For this review, take the finished solid that the model builds, in its own axes (mm). A direction names the side the tool comes from. Round coordinates to 2 decimals unless told otherwise and drop trailing zeros. Write each loop counter-clockwise with the first axis right and the second up, starting at its lowest first coordinate (ties: lowest second). Pieces come first, ordered by that corner, then holes. Notation, with made-up numbers: (20.5, 81.5) - (79.5, 81.5) arc R29 cw to (79.5, 116.5) - close; hole circle Ø7 at (81, 61). An arc over 180 degrees is marked (long way). Answer in a Markdown table with one row per item. Add a question column.
from build123d import *

# Parameters (mm, degrees)
SKETCH1_W                  = 120
SKETCH1_H                  = 80
BOSS_EXTRUDE1_DEPTH        = 15
SKETCH2_R                  = 33
BOSS_EXTRUDE2_DEPTH        = 48
BOSS_EXTRUDE3_DEPTH        = 15
SKETCH10_R                 = 21
CUT_EXTRUDE1_DEPTH         = 48
SKETCH11_R                 = 16.5
CUT_EXTRUDE2_DEPTH         = 15
M12X1_5_TAPPED_HOLE1_D     = 10.5
M12X1_5_TAPPED_HOLE1_DEPTH = 15
FILLET2_R                  = 2
FILLET3_R                  = 10


with BuildPart() as part:
    # Sketch1 → Boss-Extrude1 (new body)
    with BuildSketch(Plane(origin=(0, 0, 0), x_dir=(1, 0, 0), z_dir=(0, 1, 0))):
        Rectangle(SKETCH1_W, SKETCH1_H)
    extrude(amount=BOSS_EXTRUDE1_DEPTH)

    # Sketch2 → Boss-Extrude2 (add)
    with BuildSketch(Plane(origin=(0, 0, 0), x_dir=(1, 0, 0), z_dir=(0, 1, 0))):
        with Locations(Location((0, 0, 0), (0, 0, 270))):
            Circle(SKETCH2_R)
    extrude(amount=BOSS_EXTRUDE2_DEPTH)

    # Sketch3 → Boss-Extrude3 (add)
    with BuildSketch(Plane(origin=(0, 48, 0), x_dir=(1, 0, 0), z_dir=(0, 1, 0))):
        with BuildLine():
            ThreePointArc((-56.391046334, 10.447445772), (0, 36), (56.391046334, 10.447445772))
            ThreePointArc((56.391046334, 10.447445772), (59.733253975, 0), (56.391046334, -10.447445772))
            ThreePointArc((56.391046334, -10.447445772), (0, -36), (-56.391046334, -10.447445772))
            ThreePointArc((-56.391046334, -10.447445772), (-59.733253975, 0), (-56.391046334, 10.447445772))
        make_face()
    extrude(amount=BOSS_EXTRUDE3_DEPTH)

    # Sketch10 → Cut-Extrude1 (cut)
    with BuildSketch(Plane(origin=(0, 63, 0), x_dir=(1, 0, 0), z_dir=(0, 1, 0))):
        with Locations(Location((0, 0, 0), (0, 0, 270))):
            Circle(SKETCH10_R)
    extrude(amount=-CUT_EXTRUDE1_DEPTH, mode=Mode.SUBTRACT)

    # Sketch11 → Cut-Extrude2 (cut)
    with BuildSketch(Plane(origin=(0, 15, 0), x_dir=(1, 0, 0), z_dir=(0, 1, 0))):
        with Locations(Location((0, 0, 0), (0, 0, 270))):
            Circle(SKETCH11_R)
    extrude(amount=-CUT_EXTRUDE2_DEPTH, mode=Mode.SUBTRACT)

    # M12x1.5 Tapped Hole1
    with Locations(Plane(origin=(-42, 63, 0), x_dir=(0, 0, 1), z_dir=(0, 1, 0))):
        with Locations((0, 0), (0, 84)):
            Hole(M12X1_5_TAPPED_HOLE1_D / 2, depth=M12X1_5_TAPPED_HOLE1_DEPTH)

    # Fillet2
    fillet2_edges = [part.edges().sort_by_distance(p)[0] for p in [
        (0, 15, -33),
        (0, 48, -33),
    ]]
    fillet(fillet2_edges, radius=FILLET2_R)

    # Fillet3
    fillet3_edges = [part.edges().sort_by_distance(p)[0] for p in [
        (60, 7.5, 40),
        (-60, 7.5, 40),
        (-60, 7.5, -40),
        (60, 7.5, -40),
    ]]
    fillet(fillet3_edges, radius=FILLET3_R)


solid = part.part
Q1. To check wall thickness, follow probe 1 along X at (y, z) = (42.5, 0); probe 2 along Y at (x, z) = (48, 4); probe 3 along X at (y, z) = (9.25, 0). State the ranges of each line that lie inside material, in increasing order.
Q2. Tool access review of faces 5 (the face through (-11, 15, -13)), 6 (the face through (0.893, 55.395, 35.995)), 7 (the face through (59.733, 55.395, -0.156)): name each direction out of +Z, -Z, +X, -X, +Y, -Y from which nothing blocks a thin tool from reaching the whole face with its end or side.
Q3. Add section D-D on z = 0.5. Count the separate pieces of the cut face and the enclosed holes in it, then the cut area to 3 significant figures.
Q4. Insertion check: pin 1 Ø6 at (x, y) = (45.5, 52.5) entering from -Z; pin 2 Ø5 at (y, z) = (52.5, 16) entering from +X; pin 3 Ø6.5 at (x, z) = (-42, 0) entering from +Y. Each pin has a flat end and moves straight along its axis. Give the tip position at first contact, or say it passes through.
Q5. Add section B-B on x = -42. State the section outline as (y, z) points, then the cut area to 3 significant figures.
Q6. Add section A-A on x = 0. State the section outline as (y, z) points, then the cut area to 3 significant figures.
Q7. Draft analysis for pull direction Z (two halves, no side actions). For faces 1 (the face through (-36.795, 55.395, 0.683)), 2 (the face through (-1, 7, 40)), 3 (the face through (6.31, 39.34, 20.03)), 4 (the face through (-57.15, 7.6, -36.99)), state which applies: released by +Z, released by -Z, zero draft, split by the parting line, or undercut.
Q8. Add section C-C on y = 20. State the section outline as (x, z) points, then the cut area to 3 significant figures.
Answer sheet:
| question | item | result |
|---|---|---|
| 1 | probe 1 | x = -33 to -21, 21 to 33 |
| 1 | probe 2 | y = 0 to 15, 48 to 63 |
| 1 | probe 3 | x = -60 to -16.5, 16.5 to 60 |
| 2 | face 5 | +Y |
| 2 | face 6 | +Z, +Y |
| 2 | face 7 | +X, +Y |
| 3 | separate pieces | 4 |
| 3 | enclosed holes | 0 |
| 3 | area | 2,950 mm² |
| 4 | pin 1 | stops at z = -22.8 |
| 4 | pin 2 | stops at x = 53.56 |
| 4 | pin 3 | stops at y = 15 |
| 5 | outline | (0, -40) - (15, -40) - (15, 40) - (0, 40) - close; (48, -23.14) - (63, -23.14) - (63, -5.25) - (48, -5.25) - close; (48, 5.25) - (63, 5.25) - (63, 23.14) - (48, 23.14) - close |
| 5 | area | 1,740 mm² |
| 6 | outline | (0, -40) - (15, -40) - (15, -35) arc R2 cw to (17, -33) - (46, -33) arc R2 cw to (48, -35) - (48, -36) - (63, -36) - (63, -21) - (15, -21) - (15, -16.5) - (0, -16.5) - close; (0, 16.5) - (15, 16.5) - (15, 21) - (63, 21) - (63, 36) - (48, 36) - (48, 35) arc R2 cw to (46, 33) - (17, 33) arc R2 cw to (15, 35) - (15, 40) - (0, 40) - close |
| 6 | area | 1,950 mm² |
| 7 | face 1 | undercut |
| 7 | face 2 | released by +Z |
| 7 | face 3 | undercut |
| 7 | face 4 | released by -Z |
| 8 | outline | circle Ø66 at (0, 0); hole circle Ø42 at (0, 0) |
| 8 | area | 2,040 mm² |
